Build history of the part. All positions in model axes, mm. Round coordinates to 2 decimals unless told otherwise and drop trailing zeros. Write each loop counter-clockwise with the first axis right and the second up, starting at its lowest first coordinate (ties: lowest second). Pieces come first, ordered by that corner, then holes.
1) Saw through at B-B (y = 17.5). Write the cut outline in (x, z), plus the area to 3 significant figures.
2) Wall check: probe 1 along X at (y, z) = (-10, 22); probe 2 along X at (y, z) = (-7.5, 3). Give the ranges that are in metal, low to high.
3) Flat gauge pins, fed straight in: pin 1 (5 mm diameter, centred on y = 0, z = -10, fed in from +X); pin 2 (3 mm diameter, centred on y = -11, z = 9.5, fed in from +X); pin 3 (12 mm diameter, centred on y = -19, z = -34, fed in from -X). Where does each tip first touch, or does it go through?
4) Saw through at A-A (z = 5). Write the cut outline in (x, y).
from build123d import *

# Parameters (mm, degrees)
F0_W        = 50
F0_H        = 100
F1_DEPTH    = 819.225
F3_DEPTH    = 50.001
F4_T1_DEPTH = 327.5939866368
F4_T3_DEPTH = 327.5939866368
F5_T1_DEPTH = 329.2426603123
F5_T3_DEPTH = 329.2426603123


# Not quite as in the source:
# - a fillet or chamfer that OpenCascade refuses, or shapes differently, is made with other operations: its cross-section is extruded or revolved along the edge and cut away or added


with BuildPart() as f1:
    # F0 (on Right) → F1 (new body, symmetric)
    with BuildSketch(Plane.YZ):
        Rectangle(F0_W, F0_H)
    extrude(amount=F1_DEPTH, both=True)

    # F2 (on face) → F3 (cut, through all)
    with BuildSketch(Plane.XZ.offset(25)):
        Polygon((819.225, -50), (819.225, 50), (790.5504614241, -50), align=None)
        Polygon((-786.1531619925, -50), (-819.225, 50), (-819.225, -50), align=None)
    extrude(amount=-F3_DEPTH, mode=Mode.SUBTRACT)

    # F4: chamfer of 43.3 x 31.4592914626 on 2 edges, made by hand

    # F4_s2 → F4_t1 (cut)
    with BuildSketch(Plane(origin=(106.3006816601, 0, 370.7145326115), x_dir=(0, 1, 0), z_dir=(-0.2756373558, 0, -0.9612616959))):
        Polygon((-25, 730.4077450642), (6.4592914626, 773.7077450642), (-25, 773.7077450642), align=None)
    extrude(amount=F4_T1_DEPTH, mode=Mode.SUBTRACT)

    # F4_s4 → F4_t3 (cut)
    with BuildSketch(Plane(origin=(16.003541402, 0, 55.8109814378), x_dir=(0, 1, 0), z_dir=(0.2756373558, 0, 0.9612616959))):
        Polygon((-6.4592914626, -773.7077450642), (25, -730.4077450642), (25, -773.7077450642), align=None)
    extrude(amount=F4_T3_DEPTH, mode=Mode.SUBTRACT)

    # F5: chamfer of 43.3 x 26.721749628 on 2 edges, made by hand

    # F5_s2 → F5_t1 (cut)
    with BuildSketch(Plane(origin=(-130.827985574, 0, 395.5872834902), x_dir=(0, 1, 0), z_dir=(0.313992456, 0, -0.9494254776))):
        Polygon((-1.721749628, -762.0934641228), (25, -718.7934641228), (25, -762.0934641228), align=None)
    extrude(amount=F5_T1_DEPTH, mode=Mode.SUBTRACT)

    # F5_s4 → F5_t3 (cut)
    with BuildSketch(Plane(origin=(-27.4482740533, 0, 82.9959134631), x_dir=(0, 1, 0), z_dir=(-0.313992456, 0, 0.9494254776))):
        Polygon((-25, 718.7934641228), (1.721749628, 762.0934641228), (-25, 762.0934641228), align=None)
    extrude(amount=F5_T3_DEPTH, mode=Mode.SUBTRACT)


solid = f1.part
Evaluation:
1. outline: (-786.42, 50) - (-753.35, -50) - (756.24, -50) - (784.92, 50) - close
1. area: 154,000 mm2
2. probe 1: x = -789.96 to 787.63
2. probe 2: x = -787.94 to 785.76
3. pin 1: stops at x = 793.49
3. pin 2: stops at x = 784.8
3. pin 3: stops at x = -766.51
4. outline: (-801.4, 0) - (-758.74, -25) - (761.28, -25) - (797.07, 0) - (761.28, 25) - (-758.74, 25) - close
